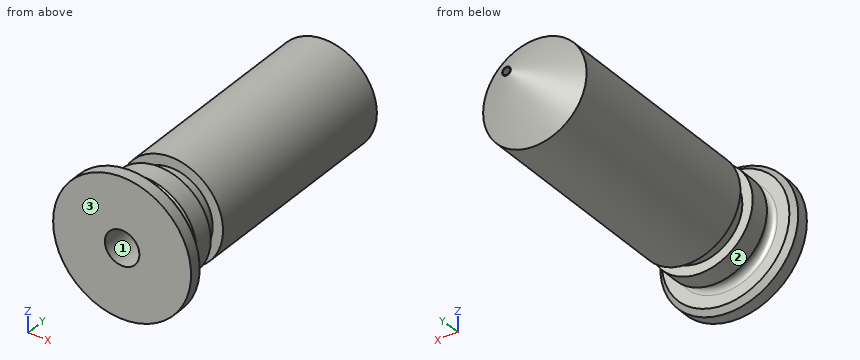
Autodesk Inventor part; units mm, degrees
ref_plane "XZ Plane" through (0, 0, 0) normal (0, 1, 0) x (-1, 0, 0)
sketch "Sketch1" plane through (0, 0, 0) normal (0, 1, 0) x (-1, 0, 0)
  circle A0 centre (0, 0) radius 4
  dimension "d0" = 8
extrude "Extrusion1" add sketch "Sketch1" along normal blind 1
sketch "Sketch2" plane through (0, 1, 0) normal (0, 1, 0) x (1, 0, 0)
  circle A0 centre (0, 0) radius 4
  circle A1 centre (0, 0) radius 3
  dimension "d3" = 6
extrude "Extrusion2" add sketch "Sketch2" along normal blind 15.5 contours A1
sketch "Sketch3" plane through (0, 0, 0) normal (0, -1, 0) x (1, 0, 0)
  circle A0 centre (0, 0) radius 4
  circle A1 centre (0, 0) radius 1
  dimension "d6" = 2
extrude "Extrusion3" cut sketch "Sketch3" against normal blind 21 contours A1
sketch "Sketch4" plane through (0, 0, 0) normal (1, 0, 0) x (0, 1, 0)
  line L0 (1, 3) -> (16.5, 3)
  line L1 (1, -3) -> (16.5, -3)
  line L2 (0, 0) -> (17, 0)
  line L3 (16.5, 3) -> (18.8075, 0.25)
  line L4 (16.5, -3) -> (16.5, 3)
  line L5 (16.5, 0.2) -> (18.8075, 0.2)
  line L6 (17.8856, 0.2) -> (16.5, 1)
  line L7 (0, 1) -> (16.5, 1)
  line L8 (16.5, 1) -> (16.5, 3)
  line L9 (18.8075, 0.25) -> (18.8075, 0.2)
  dimension "d9" = 40
  dimension "d10" = 0.2
  dimension "d11" = 30
  dimension "d20" = 0.05
revolve "Revolution1" add sketch "Sketch4" angle 360 about axis through (0, 0, 0) along (0, 1, 0) contours L3 L9 L5 L6 L4
sketch "Sketch5" plane through (0, 0, 0) normal (0, 0, 1) x (1, 0, 0)
  circle A0 centre (3, 1.35) radius 0.35
  line L0 (4, 1) -> (-4, 1)
  line L1 (3, 3) -> (3, 0)
  line L2 (0, 1.1204) -> (0, 3)
  line L3 (2.7525, 1.5975) -> (3.3734, 2.2184)
  line L4 (3.3734, 2.2184) -> (3.3499, 1.3406)
  point P0 (0, 0)
  dimension "d14" = 0.7
  dimension "d19" = 45
revolve "Revolution2" cut sketch "Sketch5" angle 360 about axis through (0, 1.1204, 0) along (0, 1, 0)
chamfer "Chamfer1" distance 0.3 angle 45 1 edges at (4, 1, 0)
sketch "Sketch6" plane through (0, 0, 0) normal (1, 0, 0) x (0, 1, 0)
  line L0 (1.845, -3) -> (16.5, -3)
  line L1 (4, -3) -> (3, -3)
  line L2 (3, -3) -> (3, -2.4)
  line L3 (3, -2.4) -> (4, -2.4)
  line L4 (4, -2.4) -> (4, -3)
  line L5 (3, 3.882) -> (3, -15)
  line L6 (1.845, -3) -> (16.5, -3)
  circle A0 centre (-0.2, 0) radius 6.5
  line L7 (0, 0) -> (0.8989, 0)
  dimension "d21" = 1
  dimension "d22" = 0.6
revolve "Revolution3" cut sketch "Sketch6" angle 360 about axis through (0, 0, 0) along (0, 1, 0) contours L2 L3 L4 L0
properties material "Copper"
Could you check a few things on this model? Use its own coordinates, in mm. Face numbers are marked on the shaded views. Give positions to 0.01 mm unless a question says otherwise; leave off trailing zeros. Write each loop counter-clockwise with the first axis right and the second up, starting at its lowest first coordinate (ties: lowest second). Pieces come first, ordered by that corner, then holes. Notation, with made-up numbers: (73, -6.5) -> (104, -6.5) arc R12 cw to (104, 15.5) -> close; hole circle Ø3 at (34.5, -20.75). An arc over 180 degrees is marked (long way). Answer as CSV lines item,"result". Start each with the question number.
(1) Please list where these lines run through material, in increasing order: line 1 (X direction, y = 12, z = 0); line 2 (Y direction, x = 3.5, z = 0.75); line 3 (Y direction, x = -1.75, z = 2.25).
(2) If we section it at C-C, the plane y = 7.25: Write out the boundary of the cut face in (x, z).
(3) If we mould it in two halves opening along X, with no side actions, what happens to the marked faces 1, 2 and 3? For each: +X half, -X half, draft (parallel to the pull), parting line (faces both ways), or undercut.
(4) I'm going to push flat-ended pins straight in: pin 1 Ø1 at (y, z) = (14, 0.5) entering from +X; pin 2 Ø1.5 at (x, y) = (2, 16.5) entering from -Z; pin 3 Ø2 at (x, z) = (-1, -1.5) entering from +Y. Where does each tip first touch, or does it pass through?
Answer list:
1,line 1,"-3 to -1, 1 to 3"
1,line 2,"0 to 1"
1,line 3,"0 to 1.03, 1.7 to 3, 4 to 16.63"
2,outline,"circle Ø6 at (0, 0); hole circle Ø2 at (0, 0)"
3,face 1,"undercut"
3,face 2,"parting line"
3,face 3,"draft"
4,pin 1,"x = 3"
4,pin 2,"z = -2.73"
4,pin 3,"y = 18.34"
